Part model, mm, in its own coordinate system. Face numbers are marked on the shaded views. A direction names the side the tool comes from. Give positions to 0.01 mm unless a question says otherwise; leave off trailing zeros. Write each loop counter-clockwise with the first axis right and the second up, starting at its lowest first coordinate (ties: lowest second). Pieces come first, ordered by that corner, then holes. Notation, with made-up numbers: M 76.5,-8.5 L 80.5,-8.5 A21 ccw 80.5,13.5 Z; hole C -31.75,86.25 d10. An arc over 180 degrees is marked long. Answer as CSV lines item,"result". Start each with the question number.
1) Mould opens along X. For the marked faces 3, 4 and 5 say: pulls with the +X half, pulls with the -X half, needs draft (parallel to the pull), parting line crosses it, or undercut.
2) Wall check: line 1 along X through (y, z) = (167, 16.55); line 2 along Y through (x, z) = (156.5, 35.5); line 3 along X through (y, z) = (99.5, 29). Give the ranges that are in metal, low to high. Write a range as from..to.
3) Tool access for the marked faces 1 and 2: list every direction of +Z, -Z, +X, -X, +Y, -Y with a clear straight run to the whole face (end or side of a thin tool).
4) Slice it at C-C, the plane y = 127. Give the cut face in (x, z), plus the area to 3 significant figures.
5) Slice it at B-B, the plane x = 42. Give the cut face in (y, z).
6) Pin check, flat tips, straight feed: pin 1 Ø5.5 at (x, y) = (159.5, 179) entering from +Z; pin 2 Ø2.5 at (x, y) = (166.5, 41) entering from -Z; pin 3 Ø7 at (x, y) = (134.5, 6.5) entering from +Z; pin 4 Ø2 at (x, y) = (83.5, 41) entering from +Z. Stop position of each tip, or through.
7) Slice it at A-A, the plane x = 132.75. Give the cut face in (y, z).
Autodesk Inventor part; units mm, degrees
ref_plane "Work Plane1" through (0, 0, 15) normal (0, 0, 1) x (1, 0, 0)
ref_plane "Work Plane2" through (87.5, 0, 15) normal (-1, 0, 0) x (0, 0, 1)
ref_plane "YZ Plane" through (0, 0, 0) normal (1, 0, 0) x (0, 1, 0)
ref_plane "Work Plane1" through (0, 0, 15) normal (0, 0, 1) x (1, 0, 0)
sketch "Sketch1" plane through (0, 0, 15) normal (0, 0, 1) x (1, 0, 0)
  line L0 (0, 0) -> (175, 0)
  line L1 (175, 0) -> (175, 185)
  line L2 (175, 185) -> (0, 185)
  line L3 (0, 185) -> (0, 0)
  dimension "d7" = 175
  dimension "d8" = 185
extrude "Extrusion1" add sketch "Sketch1" along normal blind 4
sketch "Sketch2" plane through (0, 0, 19) normal (0, 0, 1) x (1, 0, 0)
  line L0 (175, 185) -> (0, 185)
  line L1 (175, 0) -> (175, 185)
  line L2 (0, 185) -> (0, 0)
  point P0 (15.5, 179)
  point P1 (9.5, 167)
  point P2 (21.5, 167)
  point P3 (159.5, 179)
  point P4 (153.5, 167)
  point P5 (165.5, 167)
  dimension "d9" = 12
  dimension "d10" = 6
  dimension "d11" = 6
  dimension "d12" = 12
  dimension "d13" = 6
  dimension "d14" = 12
  dimension "d15" = 6
  dimension "d16" = 12
  dimension "d17" = 6
  dimension "d18" = 6
  dimension "d19" = 144
  dimension "d20" = 9.5
  dimension "d21" = 9.5
hole "Hole1" at (15.5, 179, 19) at (9.5, 167, 19) at (21.5, 167, 19) at (159.5, 179, 19) at (153.5, 167, 19) at (165.5, 167, 19) direction (0, 0, -1) diameter 3.4 end through all
sketch "Sketch3" plane through (0, 0, 19) normal (0, 0, 1) x (1, 0, 0)
  circle A0 centre (153.5, 167) radius 1.7
  circle A1 centre (21.5, 167) radius 1.7
  circle A2 centre (15.5, 179) radius 1.7
  circle A3 centre (9.5, 167) radius 1.7
  circle A4 centre (159.5, 179) radius 1.7
  circle A5 centre (165.5, 167) radius 1.7
  line L0 (175, 0) -> (175, 185)
  line L1 (175, 185) -> (0, 185)
  line L2 (0, 185) -> (0, 0)
  line L3 (0, 0) -> (175, 0)
  line L4 (2, 183) -> (173, 183)
  line L5 (173, 183) -> (173, 2)
  line L6 (173, 2) -> (2, 2)
  line L7 (2, 2) -> (2, 183)
  dimension "d34" = 2
extrude "Extrusion2" add sketch "Sketch3" along normal blind 19.05 contours L3 L2 L1 L0
sketch "Sketch5" plane through (0, 0, 15) normal (0, 0, -1) x (-1, 0, 0)
  line L0 (0, 0) -> (-175, 0)
  line L1 (0, 185) -> (0, 0)
  point P0 (-8.5, 41)
  point P1 (-22.5, 41)
  dimension "d38" = 14
  dimension "d39" = 8.5
  dimension "d40" = 41
sketch "Sketch6" plane through (0, 0, 15) normal (0, -1, 0) x (1, 0, 0)
  line L0 (0, 0) -> (0, 23.05)
  point P0 (0, -15)
  point P1 (8.5, 11.525)
  point P2 (22.5, 11.525)
  point P3 (0, 11.525)
  dimension "d41" = 8.5
  dimension "d42" = 14
hole "Hole2" at (8.5, 41, 15) at (22.5, 41, 15) direction (0, 0, 1) diameter 3 end through all
hole "Hole3" at (8.5, 0, 26.525) at (22.5, 0, 26.525) direction (0, 1, 0) diameter 3 depth 2
ref_plane "Work Plane2" through (87.5, 0, 15) normal (-1, 0, 0) x (0, 0, 1)
mirror "Mirror1" about plane through (87.5, 0, 15) normal (-1, 0, 0) of "Hole2", "Hole3"
sketch "Sketch7" plane through (0, 0, 15) normal (0, -1, 0) x (1, 0, 0)
  line L0 (58.5, 17.5) -> (116.5, 17.5) construction
  line L1 (0, 23.05) -> (175, 23.05) construction
  point P0 (0, -15)
  point P1 (87.5, 17.5)
  point P2 (87.5, 23.05)
  dimension "d57" = 58
  dimension "d58" = 5.55
hole "Hole4" at (58.5, 0, 32.5) at (116.5, 0, 32.5) direction (0, 1, 0) diameter 3 depth 2
sketch "Sketch9" plane through (0, 0, 19) normal (0, 0, 1) x (1, 0, 0)
  line L0 (173, 2) -> (2, 2)
  line L1 (173, 183) -> (173, 2)
  circle A0 centre (132.75, 6.5) radius 2.5
  circle A1 centre (132.75, 6.5) radius 4.5
  line L2 (2, 2) -> (173, 2)
  line L3 (128.25, 2) -> (137.25, 2)
  line L4 (137.25, 2) -> (137.25, 6.5)
  line L5 (137.25, 6.5) -> (128.25, 6.5)
  line L6 (128.25, 6.5) -> (128.25, 2)
  line L7 (130.25, 2) -> (135.25, 2)
  line L8 (135.25, 2) -> (135.25, 6.5)
  line L9 (135.25, 6.5) -> (130.25, 6.5)
  line L10 (130.25, 6.5) -> (130.25, 2)
  point P0 (0, 0)
  point P1 (135.25, 6.5)
  point P2 (130.25, 2.7583)
  point P3 (135.25, 2.7583)
  point P4 (132.75, 2)
  dimension "d78" = 5
  dimension "d77" = 40.25
  dimension "d79" = 2
extrude "Extrusion4" add sketch "Sketch9" along normal blind 5 contours L0 L8 A1 L4 | L5 A0 A1 | A1 L8 L5 | L5 L10 A1 | A1 L10 L0 L6
chamfer "Chamfer1" distance 1.5 angle 45 16 edges at (9.5, 168.7, 19) (21.5, 168.7, 19) (15.5, 180.7, 19) (153.5, 168.7, 19) (165.5, 168.7, 19) (159.5, 180.7, 19) (8.5, 39.5, 19) (22.5, 39.5, 19) (152.5, 39.5, 19) (166.5, 39.5, 19) (8.5, 2, 28.025) (22.5, 2, 28.025) (58.5, 2, 34) (116.5, 2, 34) (152.5, 2, 28.025) (166.5, 2, 28.025)
extrude "Extrusion5" cut sketch "Sketch9" against normal blind 5 contours L0 A1 L8 | L0 L10 A1 | A1 L10 A0 L8 | L5 A0 | A0 L5
properties part number "Table Top"
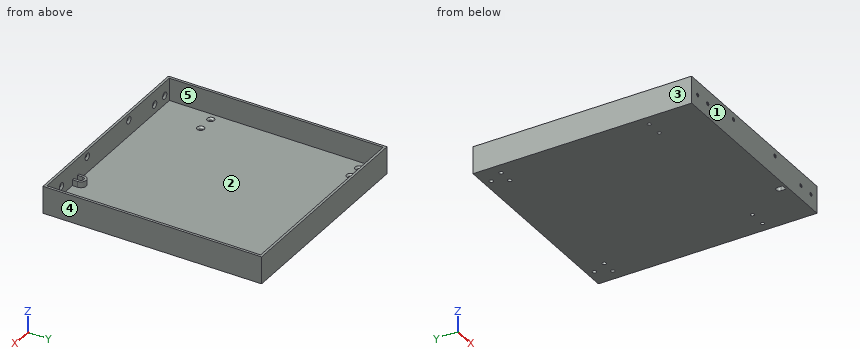
Found:
1,face 3,"pulls with the -X half"
1,face 4,"pulls with the +X half"
1,face 5,"undercut"
2,line 1,"0..7.8, 11.2..19.8, 23.2..151.8, 155.2..163.8, 167.2..175"
2,line 2,"0..2, 183..185"
2,line 3,"0..2, 173..175"
3,face 1,"+Z, -Z, +X, -X, -Y"
3,face 2,"+Z"
4,outline,"M 0,15 L 175,15 L 175,38.05 L 173,38.05 L 173,19 L 2,19 L 2,38.05 L 0,38.05 Z"
4,area,"776 mm²"
5,outline,"M 0,15 L 185,15 L 185,38.05 L 183,38.05 L 183,19 L 2,19 L 2,38.05 L 0,38.05 Z"
6,pin 1,"z = 18.55"
6,pin 2,"through"
6,pin 3,"z = 24"
6,pin 4,"z = 19"
7,outline,"M 0,15 L 2,15 L 2,38.05 L 0,38.05 Z; M 9,15 L 185,15 L 185,38.05 L 183,38.05 L 183,19 L 11,19 L 11,24 L 9,24 Z"
